Autodesk Inventor part; units mm, degrees
ref_plane "YZ Plane" through (0, 0, 0) normal (1, 0, 0) x (0, 1, 0)
ref_plane "XZ Plane" through (0, 0, 0) normal (0, 1, 0) x (-1, 0, 0)
ref_plane "XY Plane" through (0, 0, 0) normal (0, 0, 1) x (1, 0, 0)
ref_plane "Plan de construction1" through (24.857, 8.2218, -15) normal (0, 0, 1) x (0, 1, 0)
sketch "Esquisse1" plane through (24.857, 8.2218, -15) normal (0, 0, 1) x (0, 1, 0)
  circle A0 centre (-27.625, -11.5983) radius 2.25
  circle A1 centre (27.2798, -11.5983) radius 2.25
  circle A2 centre (-14.9765, -0.1949) radius 2.15
  circle A3 centre (15.0235, -0.1949) radius 2.15
  line L0 (34.7798, -18.3341) -> (-35.125, -18.3341)
  line L1 (34.7798, -4.8625) -> (34.7798, -18.3341)
  line L2 (20.0235, -4.8625) -> (34.7798, -4.8625)
  line L3 (20.0235, -4.8625) -> (20.0235, 5.1375)
  line L4 (20.0235, 5.1375) -> (11.0235, 5.1375)
  line L5 (11.0235, 5.1375) -> (11.0235, -13.773)
  line L6 (11.0235, -13.773) -> (-11.125, -13.773)
  line L7 (-11.125, -13.773) -> (-11.125, 5.1375)
  line L8 (-11.125, 5.1375) -> (-20.125, 5.1375)
  line L9 (-20.125, 5.1375) -> (-20.125, -4.8625)
  line L10 (-35.125, -4.8625) -> (-20.125, -4.8625)
  line L11 (-35.125, -18.3341) -> (-35.125, -4.8625)
  line L12 (34.7798, -18.3341) -> (-35.125, -18.3341)
  line L13 (-35.125, -18.3341) -> (-35.125, -4.8625)
  line L14 (-35.125, -4.8625) -> (34.7798, -4.8625)
  line L15 (34.7798, -4.8625) -> (34.7798, -18.3341)
  point P0 (-8.2218, 24.857)
extrude "Extrusion1" add sketch "Esquisse1" along normal blind 4 contours L0 L11 L10 L14 L7 L6 L5 L2 L1 | L5 L6 L7 L14
sketch "Esquisse2" plane through (24.857, 8.2218, -11) normal (0, 0, 1) x (1, 0, 0)
  circle A0 centre (11.5983, -27.625) radius 2.25
  circle A1 centre (11.5983, 27.2798) radius 2.25
  circle A2 centre (0.1949, -14.9765) radius 2.15
  circle A3 centre (0.1949, 15.0235) radius 2.15
  line L0 (18.3341, 34.7798) -> (18.3341, -35.125)
  line L1 (4.8625, 34.7798) -> (18.3341, 34.7798)
  line L2 (4.8625, 20.0235) -> (4.8625, 34.7798)
  line L3 (4.8625, 20.0235) -> (-5.1375, 20.0235)
  line L4 (-5.1375, 20.0235) -> (-5.1375, 11.0235)
  line L5 (-5.1375, 11.0235) -> (13.773, 11.0235)
  line L6 (13.773, 11.0235) -> (13.773, -11.125)
  line L7 (13.773, -11.125) -> (-5.1375, -11.125)
  line L8 (-5.1375, -11.125) -> (-5.1375, -20.125)
  line L9 (-5.1375, -20.125) -> (4.8625, -20.125)
  line L10 (4.8625, -35.125) -> (4.8625, -20.125)
  line L11 (18.3341, -35.125) -> (4.8625, -35.125)
  line L12 (18.3341, -35.125) -> (18.3341, 34.7798)
  line L13 (4.8625, 34.7798) -> (4.8625, -35.125)
  line L14 (18.3341, 17.5433) -> (4.8625, 17.5433)
  line L15 (4.8625, 17.5433) -> (4.8625, 13.5433)
  line L16 (4.8625, 13.5433) -> (18.3341, 13.5433)
  line L17 (18.3341, 13.5433) -> (18.3341, 17.5433)
  line L18 (18.3341, -0.1726) -> (4.8625, -0.1726) construction
  line L19 (18.3341, 13.5433) -> (18.3341, 8.5433) construction
  line L20 (18.3341, 8.5433) -> (4.8625, 8.5433)
  line L21 (4.8625, 8.5433) -> (4.8625, 4.5433)
  line L22 (4.8625, 4.5433) -> (18.3341, 4.5433)
  line L23 (18.3341, 4.5433) -> (18.3341, 8.5433)
  line L24 (4.8625, -35.125) -> (4.8625, 34.7798)
  line L25 (18.3341, -17.8886) -> (4.8625, -17.8886)
  line L26 (4.8625, -17.8886) -> (4.8625, -13.8886)
  line L27 (4.8625, -13.8886) -> (18.3341, -13.8886)
  line L28 (18.3341, -13.8886) -> (18.3341, -17.8886)
  line L29 (18.3341, -8.8886) -> (4.8625, -8.8886)
  line L30 (4.8625, -8.8886) -> (4.8625, -4.8886)
  line L31 (4.8625, -4.8886) -> (18.3341, -4.8886)
  line L32 (18.3341, -4.8886) -> (18.3341, -8.8886)
  point P0 (-24.857, -8.2218)
  dimension "d2" = 4
  dimension "d3" = 5
  dimension "d4" = 4
extrude "Extrusion2" add sketch "Esquisse2" along normal blind 10 contours L0 L16 L13 L14 | L0 L22 L6 L20 | L6 L22 L13 L20 | L0 L29 L6 L31 | L6 L29 L13 L31 | L0 L25 L13 L27
sketch "Esquisse3" plane through (29.7194, 25.7651, -11) normal (0, 1, 0) x (1, 0, 0)
  circle A0 centre (7.1312, -6) radius 2.25
  line L0 (13.4716, -10) -> (0, -10)
  point P0 (-29.7194, -11)
  dimension "d7" = 4.5
  dimension "d8" = 4
extrude "Extrusion3" cut sketch "Esquisse3" against normal blind 55.75
sketch "Esquisse4" plane through (24.857, 8.2218, -11) normal (0, 0, 1) x (1, 0, 0)
  line L0 (18.3341, 13.5433) -> (4.8625, 13.5433)
  line L1 (4.8625, 13.5433) -> (4.8625, 8.5433)
  line L2 (4.8625, 8.5433) -> (18.3341, 8.5433)
  line L3 (18.3341, 8.5433) -> (18.3341, 13.5433)
  line L4 (18.3341, -8.8886) -> (4.8625, -8.8886)
  line L5 (4.8625, -8.8886) -> (4.8625, -13.8886)
  line L6 (4.8625, -13.8886) -> (18.3341, -13.8886)
  line L7 (18.3341, -13.8886) -> (18.3341, -8.8886)
  line L8 (4.8625, 13.5433) -> (18.3341, 13.5433)
  line L9 (18.3341, 8.5433) -> (15.3341, 8.5433)
  line L10 (15.3341, 8.5433) -> (15.3341, 13.5433)
  line L11 (15.3341, 13.5433) -> (18.3341, 13.5433)
  line L12 (18.3341, 13.5433) -> (18.3341, 8.5433)
  line L13 (18.3341, -13.8886) -> (15.3341, -13.8886)
  line L14 (15.3341, -13.8886) -> (15.3341, -8.8886)
  line L15 (15.3341, -8.8886) -> (18.3341, -8.8886)
  line L16 (18.3341, -8.8886) -> (18.3341, -13.8886)
  point P0 (-24.857, -8.2218)
  dimension "d11" = 3
  dimension "d12" = 3
extrude "Extrusion4" cut sketch "Esquisse4" against normal blind 3 contours L3 L2 L10 L0 | L7 L6 L14 L4
properties part number "enclenchement"
Source: CAD feature listing. Evaluate the final solid. Frame: model axes, mm. A direction names the side the tool comes from. Give positions to 0.01 mm unless a question says otherwise; leave off trailing zeros. Order: outer loops, then holes, each group sorted by start corner. A loop starts at its lowest first (then second) coordinate and runs counter-clockwise, first axis right, second up.
(1) Pull-direction query (Y, two-part tool) for faces 6 (the face through (37, -26.903, -13)), 7 (the face through (42, -3, -14)), 8 (the face through (36, -8, -1)), 9 (the face through (36, 43.002, -13)); classes: +Y half, -Y half, draft (parallel to the pull), parting line (faces both ways), or undercut.
(2) Section query C-C (z = -5). State how many separate pieces and enclosed holes the cut face has, plus the area to 3 significant figures.
(3) Section query B-B (x = 31.75). Return the cut outline in (y, z).
(4) Section query D-D (y = 13.5). Return the cut outline in (x, z).
(5) Material intervals for line 1 along Y through (x, z) = (42.25, -5.75); line 2 along X through (y, z) = (-8.7, -5); line 3 along Y through (x, z) = (38.5, -12.75), sorted ascending.
(6) Access query for faces 1 (the face through (42, 19, -14)), 2 (the face through (36, 8, -15)), 3 (the face through (38.93, 1.36, -4.14)), 4 (the face through (36, 32, -11)), 5 (the face through (35, 3.333, -7)). Directions: +Z, -Z, +X, -X, +Y, -Y. A direction counts if a zero-diameter tool reaches every point of the face in a straight line with its end or side. Return the directions, or none.
(7) Contact query for flat-ended pins moving along their axis: P1, Ø1.5, axis at x = 33, y = 19, coming from the +Z side; P2, Ø8, axis at y = 29.5, z = -5, coming from the +X side; P3, Ø4, axis at x = 36.46, y = 35.5, coming from the -Z side; P4, Ø1.5, axis at y = 18.5, z = -12, coming from the +X side. Output: stop coordinate, or through.
(8) Section query A-A (z = -9). Return the cut outline in (x, y).
Outcome:
1. face 6: -Y half
1. face 7: undercut
1. face 8: draft
1. face 9: +Y half
2. separate pieces: 8
2. enclosed holes: 0
2. area: 144 mm2
3. outline: (-26.9, -15) - (43, -15) - (43, -11) - (25.77, -11) - (25.77, -1) - (21.77, -1) - (21.77, -11) - (16.77, -11) - (16.77, -1) - (12.77, -1) - (12.77, -11) - (3.33, -11) - (3.33, -1) - (-0.67, -1) - (-0.67, -11) - (-5.67, -11) - (-5.67, -1) - (-9.67, -1) - (-9.67, -11) - (-26.9, -11) - close
4. outline: (29.72, -15) - (43.19, -15) - (43.19, -1) - (29.72, -1) - close; hole circle Ø4.5 at (36.85, -5)
5. line 1: y = -9.67 to -5.67, -0.67 to 3.33, 12.77 to 16.77, 21.77 to 25.77
5. line 2: x = 29.72 to 34.6, 39.1 to 43.19
5. line 3: y = -26.9 to -20.34, -18.46 to 34.56, 36.44 to 43
6. face 1: +Z, +X
6. face 2: -Z, +X, -X, +Y, -Y
6. face 3: +Y, -Y
6. face 4: +Z, +X, -X, +Y
6. face 5: +Z, +X, -X
7. P1: stops at z = -11
7. P2: stops at x = 43.19
7. P3: passes through
7. P4: stops at x = 40.19
8. outline: (29.72, -9.67) - (43.19, -9.67) - (43.19, -5.67) - (29.72, -5.67) - close; (29.72, -0.67) - (43.19, -0.67) - (43.19, 3.33) - (29.72, 3.33) - close; (29.72, 12.77) - (43.19, 12.77) - (43.19, 16.77) - (29.72, 16.77) - close; (29.72, 21.77) - (43.19, 21.77) - (43.19, 25.77) - (29.72, 25.77) - close
